```python
from build123d import *

# Parameters (mm, degrees)
SKETCH1_R           = 4.5
SKETCH1_R_2         = 0.85
SKETCH1_R_3         = 1.55
BOSS_EXTRUDE2_DEPTH = 8
SKETCH5_R           = 8.2
CUT_EXTRUDE3_DEPTH  = 5
SKETCH6_R           = 3.5
CUT_EXTRUDE6_DEPTH  = 2


with BuildPart() as part:
    # Sketch1 → Boss-Extrude2 (new body)
    with BuildSketch(Plane.XY):
        with BuildLine():
            Line((-35, 4.5), (-25, 4.5))
            ThreePointArc((-25, 4.5), (-17.961764947, 17.961764947), (-4.5, 25))
            Line((-4.5, 25), (-4.5, 35))
            ThreePointArc((-4.5, 35), (0, 39.5), (4.5, 35))
            Line((4.5, 35), (4.5, 25))
            ThreePointArc((4.5, 25), (17.961764947, 17.961764947), (25, 4.5))
            Line((25, 4.5), (35, 4.5))
            ThreePointArc((35, 4.5), (39.5, 0), (35, -4.5))
            Line((35, -4.5), (25, -4.5))
            ThreePointArc((25, -4.5), (17.961764947, -17.961764947), (4.5, -25))
            Line((4.5, -25), (4.5, -35))
            ThreePointArc((4.5, -35), (0, -39.5), (-4.5, -35))
            Line((-4.5, -35), (-4.5, -25))
            ThreePointArc((-4.5, -25), (-17.961764947, -17.961764947), (-25, -4.5))
            Line((-25, -4.5), (-35, -4.5))
            ThreePointArc((-35, -4.5), (-39.5, 0), (-35, 4.5))
        make_face()
        Circle(SKETCH1_R, mode=Mode.SUBTRACT)
        with Locations((8.980256121, 8.980256121)):
            Circle(SKETCH1_R_2, mode=Mode.SUBTRACT)
        with Locations((8.980256121, -8.980256121)):
            Circle(SKETCH1_R_2, mode=Mode.SUBTRACT)
        with Locations((-8.980256121, -8.980256121)):
            Circle(SKETCH1_R_2, mode=Mode.SUBTRACT)
        with Locations((-8.980256121, 8.980256121)):
            Circle(SKETCH1_R_2, mode=Mode.SUBTRACT)
        with Locations((-35, 0)):
            Circle(SKETCH1_R_3, mode=Mode.SUBTRACT)
        with Locations((0, 35)):
            Circle(SKETCH1_R_3, mode=Mode.SUBTRACT)
        with Locations((35, 0)):
            Circle(SKETCH1_R_3, mode=Mode.SUBTRACT)
        with Locations((0, -35)):
            Circle(SKETCH1_R_3, mode=Mode.SUBTRACT)
    extrude(amount=BOSS_EXTRUDE2_DEPTH)

    # Sketch5 → Cut-Extrude3 (cut)
    with BuildSketch(Plane(origin=(0, 0, 0), x_dir=(-1, 0, 0), z_dir=(0, 0, -1))):
        Circle(SKETCH5_R)
    extrude(amount=-CUT_EXTRUDE3_DEPTH, mode=Mode.SUBTRACT)

    # Sketch6 → Cut-Extrude6 (cut)
    with BuildSketch(Plane.XY):
        with Locations((0, 35)):
            Circle(SKETCH6_R)
        with Locations((35, 0)):
            Circle(SKETCH6_R)
        with Locations((0, -35)):
            Circle(SKETCH6_R)
        with Locations((-35, 0)):
            Circle(SKETCH6_R)
    extrude(amount=CUT_EXTRUDE6_DEPTH, mode=Mode.SUBTRACT)


solid = part.part
```
Input: part model. Units: mm. Frame: model coordinates. A direction names the side the tool comes from. Coordinates: 2 decimals unless noted, no trailing zeros. Loops run counter-clockwise (first coordinate to the right, second up) from the corner with the lowest first, then second, coordinate; pieces in that order, holes last. Notation, with made-up numbers: M 6.25,32.5 L 34.25,32.5 A18 cw 34.25,62.5 Z; hole C 79,-34 d1. An arc over 180 degrees is marked long. One line per item, written item: value.
(1) Pull-direction query (X, two-part tool) for faces 5 (the cylindrical face through (0.1, -39.5, 3.9)), 6 (the flat face through (30, -4.5, 4)), 7 (the cylindrical face through (-9.83, -8.94, 3.94)); classes: +X half, -X half, draft (parallel to the pull), parting line (faces both ways), or undercut.
Filled in:
face 5: parting line
face 6: draft
face 7: undercut
(2) Pin query (flat end, axial travel): pin 1 (2 mm diameter, centred on y = -13, z = 4.5, fed in from -X); pin 2 (2 mm diameter, centred on x = -15.5, z = 4.5, fed in from +Y); pin 3 (5 mm diameter, centred on x = -2.5, y = 2, fed in from -Z). Return the tip coordinate at first contact, or that it passes through.
Filled in:
pin 1: x = -22.39
pin 2: y = 20.86
pin 3: z = 5
(3) Section A-A (y = 0). Output: boundary loops of the cut face in (x, z), and give its area (3 significant figures).
Filled in:
outline: M -39.5,0 L -38.5,0 L -38.5,2 L -36.55,2 L -36.55,8 L -39.5,8 Z; M -33.45,2 L -31.5,2 L -31.5,0 L -8.2,0 L -8.2,5 L -4.5,5 L -4.5,8 L -33.45,8 Z; M 4.5,5 L 8.2,5 L 8.2,0 L 31.5,0 L 31.5,2 L 33.45,2 L 33.45,8 L 4.5,8 Z; M 36.55,2 L 38.5,2 L 38.5,0 L 39.5,0 L 39.5,8 L 36.55,8 Z
area: 458 mm^2
(4) Reachability of faces 1 (the flat face through (30, 4.5, 4)), 2 (the flat face through (-4.5, 30, 4)), 3 (the flat face through (-30, -4.5, 4)), 4 (the flat face through (2, -36, 2)) from +Z, -Z, +X, -X, +Y, -Y: full face, straight path, thin tool, end or side. Return the list, or none.
Filled in:
face 1: +Z, -Z, +X, +Y
face 2: +Z, -Z, -X, +Y
face 3: +Z, -Z, -X, -Y
face 4: -Z
(5) Section D-D (y = 21). Output: boundary loops of the cut face in (x, z), and give its area (3 significant figures).
Filled in:
outline: M -14.29,0 L 14.29,0 L 14.29,8 L -14.29,8 Z
area: 229 mm^2
(6) Section C-C (x = -26). Output: boundary loops of the cut face in (y, z).
Filled in:
outline: M -4.5,0 L 4.5,0 L 4.5,8 L -4.5,8 Z
(7) Line query: line 1 along Y through (x, z) = (0, 6.35); line 2 along Y through (x, z) = (0, 0.95); line 3 along X through (y, z) = (-9, 7.5). Output: solid intervals per line, ascending. Write a range as from..to.
Filled in:
line 1: -39.5..-36.55, -33.45..-4.5, 4.5..33.45, 36.55..39.5
line 2: -39.5..-38.5, -31.5..-8.2, 8.2..31.5, 38.5..39.5
line 3: -23.75..-9.83, -8.13..8.13, 9.83..23.75
